Design review of the part built by this model. Coordinates are the model's own, in mm. Face numbers are marked on the shaded views. A direction names the side the tool comes from. Give positions to 0.01 mm unless a question says otherwise; leave off trailing zeros. Loops run counter-clockwise (first coordinate to the right, second up) from the corner with the lowest first, then second, coordinate; pieces in that order, holes last. Notation, with made-up numbers: (29, 79.5) -> (74, 79.5) arc R20 ccw to (74, 117.5) -> close; hole circle Ø1 at (-40, 47). An arc over 180 degrees is marked (long way). Use a Markdown table: item, result. Add a question column.
1. Add section D-D (y = -25). State the section outline as (x, z) points.
2. For the marked faces 1 and 2, list the 3-axis set-ups (+Z, -Z, +X, -X, +Y, -Y) from which the entire face can be reached by the end or side of a thin tool; tool diameter is ignored.
3. Draft analysis for pull direction X (two halves, no side actions). For the marked faces 3, 4 and 5, state which applies: pulls with the +X half, pulls with the -X half, needs draft (parallel to the pull), parting line crosses it, or undercut.
4. Add section A-A (z = 1.75). Count the separate pieces of the cut face and the enclosed holes in it, and give its area (3 significant figures).
5. To check wall thickness, follow line 1 (Y direction, x = 30.5, z = 8.75); line 2 (X direction, y = -51, z = 10); line 3 (Y direction, x = 34, z = 6.5). State the ranges of each line that lie inside material, in increasing order.
6. Add section C-C (x = 20.5). State the section outline as (y, z) points, and give its area (3 significant figures).
7. For pin 1 Ø0.6 at (x, y) = (26, -4.5) entering from -Z; pin 2 Ø7 at (x, y) = (30.5, -4) entering from -Z, all flat-tipped, find the tip position at first contact; note any pin that passes through.
8. Add section B-B (y = -51). State the section outline as (x, z) points, and give its area (3 significant figures).
```python
from build123d import *

# Parameters (mm, degrees)
F0_W     = 20
F0_H     = 8
F1_DEPTH = 12
F2_DEPTH = 5
F3_DEPTH = 5
F5_DEPTH = 2
F4_R     = 2.25
F6_DEPTH = 25
F8_DEPTH = 2
F7_R     = 2.25
F9_DEPTH = 25


with BuildPart() as f1:
    # F0 (on Top) → F1 (new body)
    with BuildSketch(Plane.XY):
        with Locations((25.5, -4)):
            Rectangle(F0_W, F0_H)
        with Locations((25.5, -51)):
            Rectangle(F0_W, F0_H)
        with BuildLine():
            Line((6, 0), (0, 0))
            Line((0, 0), (0, -55))
            Line((0, -55), (6, -55))
            Line((6, -55), (6, -45.71))
            ThreePointArc((6, -45.71), (3.75, -43.46), (6, -41.21))
            Line((6, -41.21), (6, -32.98))
            ThreePointArc((6, -32.98), (3.75, -30.73), (6, -28.48))
            Line((6, -28.48), (6, -20.25))
            ThreePointArc((6, -20.25), (3.75, -18), (6, -15.75))
            Line((6, -15.75), (6, -7.52))
            ThreePointArc((6, -7.52), (3.75, -5.27), (6, -3.02))
            Line((6, -3.02), (6, 0))
        make_face()
        with BuildLine():
            Line((51, 0), (45, 0))
            Line((45, 0), (45, -3.02))
            ThreePointArc((45, -3.02), (46.5909902577, -3.6790097423), (47.25, -5.27))
            ThreePointArc((47.25, -5.27), (46.5909902577, -6.8609902577), (45, -7.52))
            Line((45, -7.52), (45, -15.75))
            ThreePointArc((45, -15.75), (46.5909902577, -16.4090097423), (47.25, -18))
            ThreePointArc((47.25, -18), (46.5909902577, -19.5909902577), (45, -20.25))
            Line((45, -20.25), (45, -28.48))
            ThreePointArc((45, -28.48), (46.5909902577, -29.1390097423), (47.25, -30.73))
            ThreePointArc((47.25, -30.73), (46.5909902577, -32.3209902577), (45, -32.98))
            Line((45, -32.98), (45, -41.21))
            ThreePointArc((45, -41.21), (46.5909902577, -41.8690097423), (47.25, -43.46))
            ThreePointArc((47.25, -43.46), (46.5909902577, -45.0509902577), (45, -45.71))
            Line((45, -45.71), (45, -55))
            Line((45, -55), (51, -55))
            Line((51, -55), (51, 0))
        make_face()
        with BuildLine():
            Line((15.5, 0), (6, 0))
            Line((6, 0), (6, -3.02))
            ThreePointArc((6, -3.02), (7.5909902577, -3.6790097423), (8.25, -5.27))
            ThreePointArc((8.25, -5.27), (7.5909902577, -6.8609902577), (6, -7.52))
            Line((6, -7.52), (6, -15.75))
            ThreePointArc((6, -15.75), (7.5909902577, -16.4090097423), (8.25, -18))
            ThreePointArc((8.25, -18), (7.5909902577, -19.5909902577), (6, -20.25))
            Line((6, -20.25), (6, -28.48))
            ThreePointArc((6, -28.48), (7.5909902577, -29.1390097423), (8.25, -30.73))
            ThreePointArc((8.25, -30.73), (7.5909902577, -32.3209902577), (6, -32.98))
            Line((6, -32.98), (6, -41.21))
            ThreePointArc((6, -41.21), (7.5909902577, -41.8690097423), (8.25, -43.46))
            ThreePointArc((8.25, -43.46), (7.5909902577, -45.0509902577), (6, -45.71))
            Line((6, -45.71), (6, -55))
            Line((6, -55), (15.5, -55))
            Line((15.5, -55), (15.5, -47))
            Line((15.5, -47), (15.5, -8))
            Line((15.5, -8), (15.5, 0))
        make_face()
        with BuildLine():
            Line((45, 0), (35.5, 0))
            Line((35.5, 0), (35.5, -8))
            Line((35.5, -8), (35.5, -47))
            Line((35.5, -47), (35.5, -55))
            Line((35.5, -55), (45, -55))
            Line((45, -55), (45, -45.71))
            ThreePointArc((45, -45.71), (42.75, -43.46), (45, -41.21))
            Line((45, -41.21), (45, -32.98))
            ThreePointArc((45, -32.98), (42.75, -30.73), (45, -28.48))
            Line((45, -28.48), (45, -20.25))
            ThreePointArc((45, -20.25), (42.75, -18), (45, -15.75))
            Line((45, -15.75), (45, -7.52))
            ThreePointArc((45, -7.52), (42.75, -5.27), (45, -3.02))
            Line((45, -3.02), (45, 0))
        make_face()
    extrude(amount=F1_DEPTH)

    # F0 (on Top) → F2 (cut)
    with BuildSketch(Plane.XY):
        with Locations((25.5, -51)):
            Rectangle(F0_W, F0_H)
    extrude(amount=F2_DEPTH, mode=Mode.SUBTRACT)

    # F0 (on Top) → F3 (cut)
    with BuildSketch(Plane.XY):
        with Locations((25.5, -4)):
            Rectangle(F0_W, F0_H)
    extrude(amount=F3_DEPTH, mode=Mode.SUBTRACT)

    # F4 (on face) → F5 (cut)
    with BuildSketch(Plane(origin=(0, 0, 5), x_dir=(1, 0, 0), z_dir=(0, 0, -1))):
        Polygon((24.5, 47), (25.5, 47), (26.5, 47), (26.5, 52), (24.5, 52), align=None)
    extrude(amount=-F5_DEPTH, mode=Mode.SUBTRACT)

    # F4 (on face) → F6 (cut)
    with BuildSketch(Plane(origin=(0, 0, 5), x_dir=(1, 0, 0), z_dir=(0, 0, -1))):
        with Locations((20.5, 51)):
            Circle(F4_R)
        with Locations((30.5, 51)):
            Circle(F4_R)
    extrude(amount=-F6_DEPTH, mode=Mode.SUBTRACT)

    # F7 (on face) → F8 (cut)
    with BuildSketch(Plane(origin=(0, 0, 5), x_dir=(1, 0, 0), z_dir=(0, 0, -1))):
        Polygon((26.5, 8), (25.5, 8), (24.5, 8), (24.5, 3), (26.5, 3), align=None)
    extrude(amount=-F8_DEPTH, mode=Mode.SUBTRACT)

    # F7 (on face) → F9 (cut)
    with BuildSketch(Plane(origin=(0, 0, 5), x_dir=(1, 0, 0), z_dir=(0, 0, -1))):
        with Locations((30.5, 4)):
            Circle(F7_R)
        with Locations((20.5, 4)):
            Circle(F7_R)
    extrude(amount=-F9_DEPTH, mode=Mode.SUBTRACT)


solid = f1.part
```
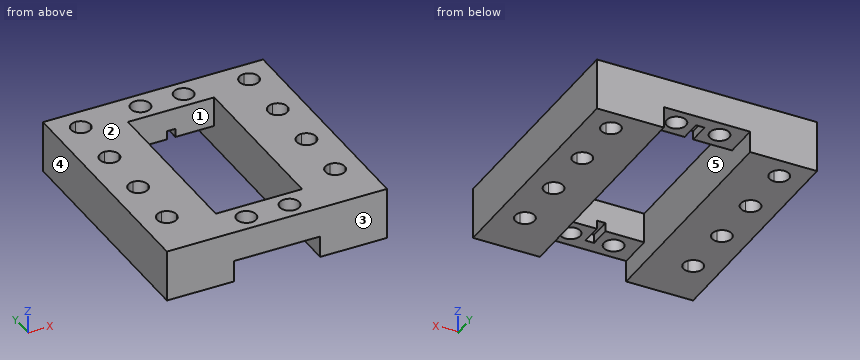
Taken from the geometry:
| question | item | result |
|---|---|---|
| 1 | outline | (0, 0) -> (15.5, 0) -> (15.5, 12) -> (0, 12) -> close; (35.5, 0) -> (51, 0) -> (51, 12) -> (35.5, 12) -> close |
| 2 | face 1 | +Z, -Z |
| 2 | face 2 | +Z, +X, -X, +Y, -Y |
| 3 | face 3 | needs draft |
| 3 | face 4 | pulls with the -X half |
| 3 | face 5 | undercut |
| 4 | separate pieces | 2 |
| 4 | enclosed holes | 8 |
| 4 | area | 1,580 mm^2 |
| 5 | line 1 | y = -55 to -53.25, -48.75 to -47, -8 to -6.25, -1.75 to 0 |
| 5 | line 2 | x = 0 to 18.25, 22.75 to 28.25, 32.75 to 51 |
| 5 | line 3 | y = -55 to -47, -8 to 0 |
| 6 | outline | (-55, 5) -> (-53.25, 5) -> (-53.25, 12) -> (-55, 12) -> close; (-48.75, 5) -> (-47, 5) -> (-47, 12) -> (-48.75, 12) -> close; (-8, 5) -> (-6.25, 5) -> (-6.25, 12) -> (-8, 12) -> close; (-1.75, 5) -> (0, 5) -> (0, 12) -> (-1.75, 12) -> close |
| 6 | area | 49.0 mm^2 |
| 7 | pin 1 | stops at z = 7 |
| 7 | pin 2 | stops at z = 5 |
| 8 | outline | (0, 0) -> (15.5, 0) -> (15.5, 5) -> (18.25, 5) -> (18.25, 12) -> (0, 12) -> close; (22.75, 5) -> (24.5, 5) -> (24.5, 7) -> (26.5, 7) -> (26.5, 5) -> (28.25, 5) -> (28.25, 12) -> (22.75, 12) -> close; (32.75, 5) -> (35.5, 5) -> (35.5, 0) -> (51, 0) -> (51, 12) -> (32.75, 12) -> close |
| 8 | area | 445 mm^2 |
